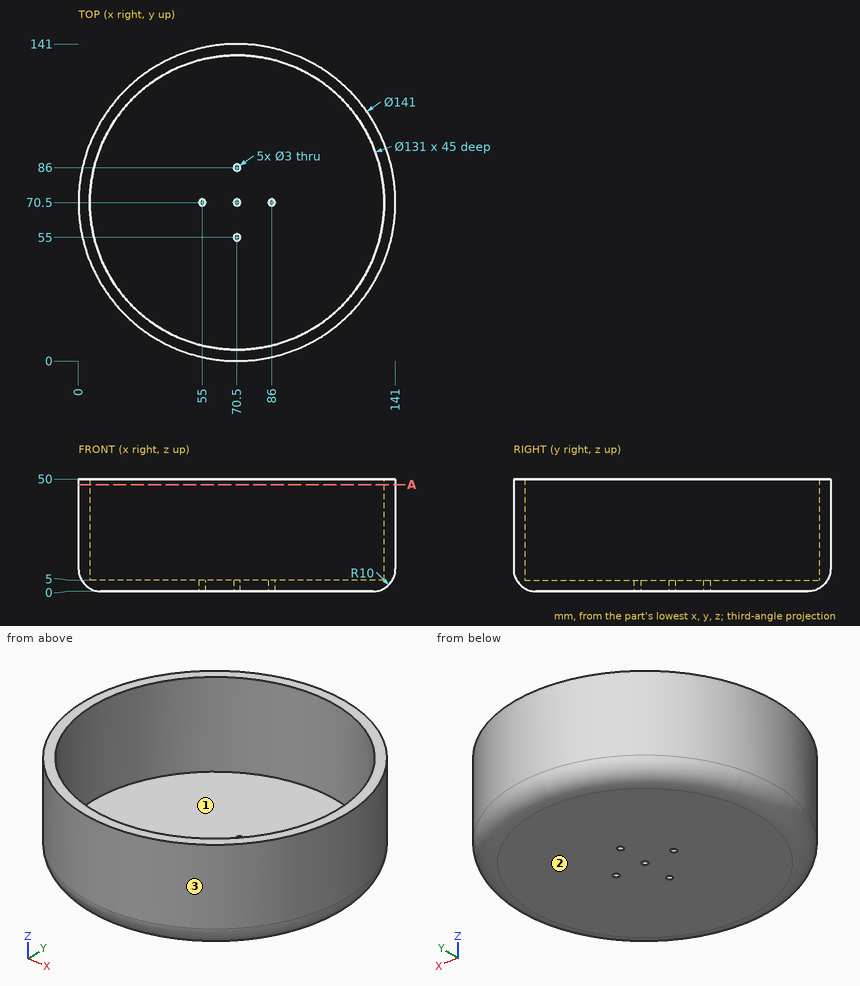
The figure shows three views and two pictorial views of one solid part (mm, origin at its lowest corner). Answer the questions. Give positions to 0.01 mm unless a question says otherwise; leave off trailing zeros. Write each loop counter-clockwise with the first axis right and the second up, starting at its lowest first coordinate (ties: lowest second). Pieces come first, ordered by that corner, then holes. Notation, with made-up numbers: (75, -31) - (129, -31) arc R25 cw to (129, 5) - close; hole circle Ø2 at (12.5, 39). An arc over 180 degrees is marked (long way). Use CSV: the item, a comma, the result in double quotes. Start each with the question number.
Item 1: Consider line 1 (Y direction, x = 86, z = 2.7); line 2 (Z direction, x = 85, y = 42); line 3 (Y direction, x = 86, z = 3.45). Determine where each line is inside the solid, lowest interval first.
Item 2: Flat-ended cylindrical pins translate along their axes: P1, Ø12, axis at x = 111, z = 5, coming from the +Y side; P2, Ø3, axis at x = 124, z = 8, coming from the -Y side; P3, Ø2.5, axis at x = 55, y = 70.5, coming from the -Z side; P4, Ø3, axis at x = 87, y = 106, coming from the -Z side. Find the tip coordinate at first contact, or state that the pin passes through.
Item 3: The part is cut by section A-A, the plane z = 47.5. Give the vertices of the cut face in (x, y).
Item 4: The mould has two halves that part along Y. Classify the marked faces 1, 2 and 3: pulls with the +Y half, pulls with the -Y half, needs draft (parallel to the pull), parting line crosses it, or undercut.
Taken from the geometry:
1,line 1,"4.97 to 69, 72 to 136.03"
1,line 2,"0 to 5"
1,line 3,"4.23 to 69, 72 to 136.77"
2,P1,"y = 131.31"
2,P2,"y = 23.14"
2,P3,"through"
2,P4,"z = 0"
3,outline,"circle Ø141 at (70.5, 70.5); hole circle Ø131 at (70.5, 70.5)"
4,face 1,"undercut"
4,face 2,"needs draft"
4,face 3,"parting line crosses it"
